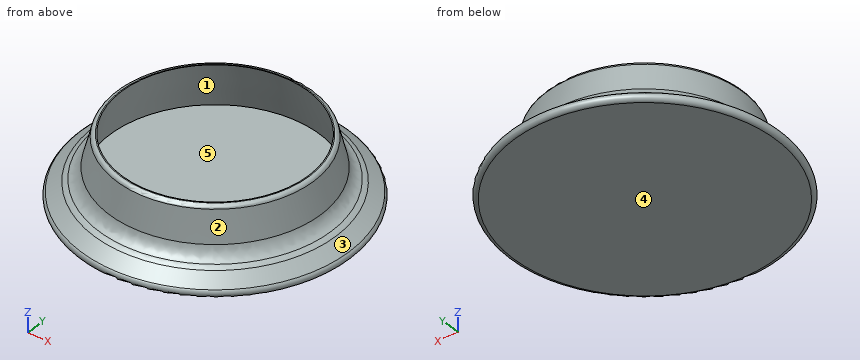
```python
from build123d import *

# Parameters (mm, degrees)
F2_T = -1.27
F3_R = 1.27
F4_R = 1.27
F5_R = 5.08


with BuildPart() as f1:
    # F0 (on Front) → F1 (revolve)
    with BuildSketch(Plane.XZ):
        with BuildLine():
            Line((0, 19.05), (0, 0))
            Line((0, 0), (43.18, 0))
            Line((43.18, 0), (36.1202941176, 5.1351804111))
            ThreePointArc((36.1202941176, 5.1351804111), (34.3489379305, 6.0386627498), (32.385, 6.35))
            Line((32.385, 6.35), (29.21, 19.05))
            Line((29.21, 19.05), (0, 19.05))
        make_face()
    revolve(axis=Axis((0, 0, 9.525), (0, 0, -1)))

    # F2
    f2_openings = [f1.faces().sort_by_distance(p)[0] for p in [
        (0, 0, 19.05),
    ]]
    offset(amount=F2_T, openings=f2_openings, kind=Kind.INTERSECTION)

    # F3
    f3_edges = [f1.edges().sort_by_distance(p)[0] for p in [
        (-43.18, 0, 0),
    ]]
    fillet(f3_edges, radius=F3_R)

    # F4
    f4_edges = [f1.edges().sort_by_distance(p)[0] for p in [
        (-29.21, 0, 19.05),
    ]]
    fillet(f4_edges, radius=F4_R)

    # F5
    f5_edges = [f1.edges().sort_by_distance(p)[0] for p in [
        (-32.385, 0, 6.35),
    ]]
    fillet(f5_edges, radius=F5_R)


solid = f1.part
```
Here's how the part is built. I have some questions about the finished solid (model axes, mm). Face numbers are marked on the shaded views. A direction names the side the tool comes from. Coordinates: 2 decimals unless noted, no trailing zeros. Order: outer loops, then holes, each group sorted by start corner. A loop starts at its lowest first (then second) coordinate and runs counter-clockwise, first axis right, second up. Notation, with made-up numbers: M 50,51 L 82,51 A12 ccw 82,60 Z; hole C 27,54 d9. An arc over 180 degrees is marked long. Answer as a JSON object with one key per item and string values. Group by question number.
(1) I need wall thicknesses on probe 1 along Z at (x, y) = (-12, -34); probe 2 along Z at (x, y) = (15, 34); probe 3 along Z at (x, y) = (20.5, -7). Which ranges of each line are inside material? Lowest first, please.
(2) Which directions (+Z, -Z, +X, -X, +Y, -Y) give clear straight access to the entire face, cutting with the end or side of a thin tool? Please do the marked faces 1 and 2.
(3) For pin 1 (6 mm diameter, centred on y = -26, z = 5.5, fed in from +X) (3 decimals); pin 2 (5 mm diameter, centred on y = -1.5, z = 17, fed in from -X); pin 3 (5 mm diameter, centred on y = 3, z = 11.5, fed in from +X); pin 4 (8 mm diameter, centred on x = -6.5, y = 22, fed in from -Z), each with a flat end and sliding along its axis, tell me the tip position at first contact or that it passes through.
(4) Suppose I cut it at A-A, the plane z = 14.5. Please give me the cut outline in (x, y) (1 decimal).
(5) If we mould it in two halves opening along X, with no side actions, what happens to the marked faces 3, 4 and 5? For each: released by +X, released by -X, zero draft, split by the parting line, or undercut.
Values found:
{
 "1": {"probe 1": "z = 0 to 1.27, 3.61 to 5.18", "probe 2": "z = 0 to 1.27, 2.81 to 4.38", "probe 3": "z = 0 to 1.27"},
 "2": {"face 1": "none", "face 2": "+Z"},
 "3": {"pin 1": "stops at x = 30.615", "pin 2": "stops at x = -30.32", "pin 3": "stops at x = 31.63", "pin 4": "stops at z = 0"},
 "4": {"outline": "C 0,0 d60.7; hole C 0,0 d58.1"},
 "5": {"face 3": "split by the parting line", "face 4": "zero draft", "face 5": "undercut"}
}
